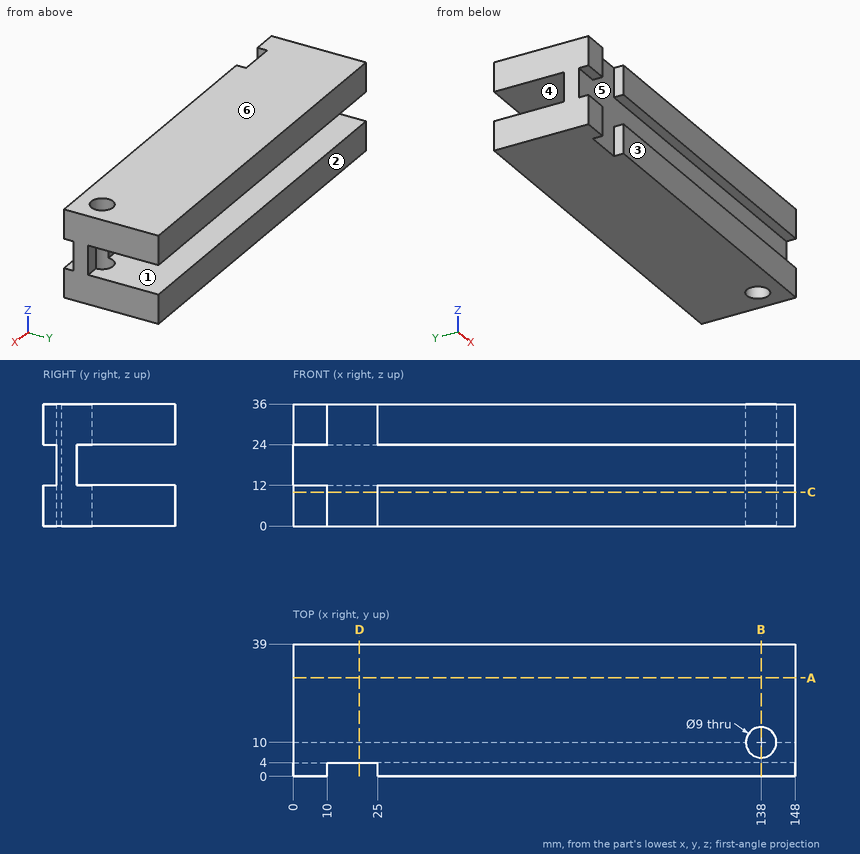
Study the drawing (mm; zero at the part's minimum x, y, z) and answer. A direction names the side the tool comes from. Coordinates: 2 decimals unless noted, no trailing zeros. Write each loop counter-clockwise with the first axis right and the second up, starting at its lowest first coordinate (ties: lowest second). Pieces come first, ordered by that corner, then holes. Notation, with made-up numbers: (-17.75, -24.75) - (5.25, -24.75) arc R8 cw to (5.25, -20.75) - close; hole circle Ø5 at (-21, 35.25). An arc over 180 degrees is marked (long way). One line per item, written item: value.
1) Find section A-A (y = 29). Give the vertices of the cut face in (x, z), and give its area (3 significant figures).
Geometry check:
outline: (0, 0) - (148, 0) - (148, 12) - (0, 12) - close; (0, 24) - (148, 24) - (148, 36) - (0, 36) - close
area: 3,550 mm2
2) Find section B-B (x = 138). Give the vertices of the cut face in (y, z), and give its area (3 significant figures).
Geometry check:
outline: (0, 0) - (5.5, 0) - (5.5, 36) - (0, 36) - (0, 24) - (4, 24) - (4, 12) - (0, 12) - close; (14.5, 0) - (39, 0) - (39, 12) - (14.5, 12) - close; (14.5, 24) - (39, 24) - (39, 36) - (14.5, 36) - close
area: 738 mm2
3) Find section C-C (z = 10). Give the vertices of the cut face in (x, y).
Geometry check:
outline: (0, 0) - (10, 0) - (10, 4) - (25, 4) - (25, 0) - (148, 0) - (148, 39) - (0, 39) - close; hole circle Ø9 at (138, 10)
4) Find section D-D (x = 19.5). Give the vertices of the cut face in (y, z), and give its area (3 significant figures).
Geometry check:
outline: (4, 0) - (39, 0) - (39, 12) - (10, 12) - (10, 24) - (39, 24) - (39, 36) - (4, 36) - close
area: 912 mm2
5) Consider line 1 along X through (y, z) = (10, 25.5); line 2 along Z through (x, y) = (47.5, 31); line 3 along Y through (x, z) = (138, 16). Determine where each line is inside the solid, lowest interval first. Write a range as from..to.
Geometry check:
line 1: x = 0..133.5, 142.5..148
line 2: z = 0..12, 24..36
line 3: y = 4..5.5
6) For a pull along Z with two mould halves and no side action, classify the marked faces 3, 4, 5 and 6 as pulls with the +Z half, pulls with the -Z half, needs draft (parallel to the pull), parting line crosses it, or undercut.
Geometry check:
face 3: needs draft
face 4: undercut
face 5: undercut
face 6: pulls with the +Z half
7) This flat-tipped pin is pushed along its axis until it touches: pin 1 Ø2 at (x, z) = (60, 17) entering from +Y. Where does it stop, or does it pass through?
Geometry check:
pin 1: stops at y = 10
8) A tool of negligible diameter and unlimited length cuts with its end or side. For the marked faces 1 and 2, from which of +Z, -Z, +X, -X, +Y, -Y can it reach the whole face along a straight path? Write none if from no direction.
Geometry check:
face 1: +X, -X, +Y
face 2: +Z, -Z, +X, -X, +Y
